For this review, take the finished solid that the model builds, in its own axes (mm). Face numbers are marked on the shaded views. A direction names the side the tool comes from. Coordinates: 2 decimals unless noted, no trailing zeros. Order: outer loops, then holes, each group sorted by start corner. A loop starts at its lowest first (then second) coordinate and runs counter-clockwise, first axis right, second up. Notation, with made-up numbers: (15.5, 71) - (27.5, 71) arc R24 cw to (27.5, 93) - close; hole circle Ø7 at (40, 58.5). An arc over 180 degrees is marked (long way). One line per item, written item: value. Start each with the question number.
(1) To check wall thickness, follow line 1 along Z through (x, y) = (190, -57); line 2 along X through (y, z) = (-8, 7); line 3 along Y through (x, z) = (220.5, 42.5). State the ranges of each line that lie inside material, in increasing order.
(2) Consider section C-C on z = 34. Write out the cut boundary in (x, y).
(3) Clearance check with flat-ended pins moving along their axes: pin 1 (4 mm diameter, centred on x = 156, y = 125, fed in from +Z); pin 2 (4 mm diameter, centred on x = 200.5, z = 49, fed in from +Y). State where each tip first meets the part, or that it passes through.
(4) Consider section D-D on y = 42. Write out the cut boundary in (x, z), then the cut area to 3 significant figures.
(5) Consider section B-B on x = 206. Write out the cut boundary in (y, z), then the cut area to 3 significant figures.
(6) Consider section A-A on y = 0. Write out the cut boundary in (x, z).
(7) For the marked faces 1, 2 and 3, list the 3-axis set-ups (+Z, -Z, +X, -X, +Y, -Y) from which the entire face can be reached by the end or side of a thin tool; tool diameter is ignored.
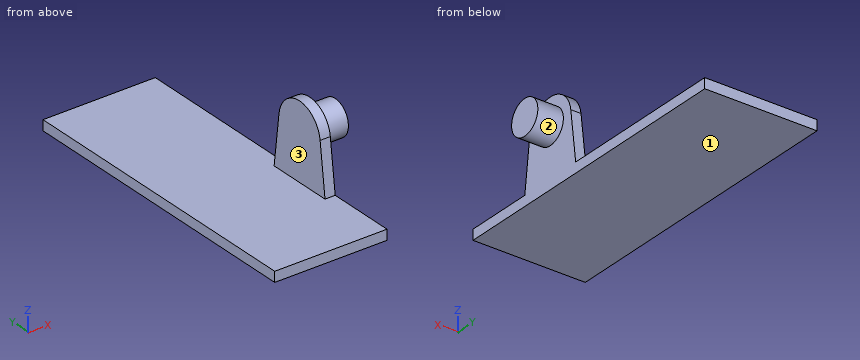
```python
from build123d import *

# Parameters (mm, degrees)
F4_W     = 110
F4_H     = 300
F5_DEPTH = 9.9999997765
F0_R     = 16.989496858
F1_DEPTH = 10
F2_DEPTH = 25


with BuildPart() as f5:
    # F4 (on Top) → F5 (new body)
    with BuildSketch(Plane.XY):
        with Locations((155, 50)):
            Rectangle(F4_W, F4_H)
    extrude(amount=-F5_DEPTH)

    # F0 (on face) → F1 (join)
    with BuildSketch(Plane.YZ.offset(210)):
        with BuildLine():
            ThreePointArc((26.601998421, 49.9582877529), (0, 73.3968899806), (-26.601998421, 49.9582877529))
            Line((-26.601998421, 49.9582877529), (-32.9437274149, 0))
            Line((-32.9437274149, 0), (32.9437274149, 0))
            Line((32.9437274149, 0), (26.601998421, 49.9582877529))
        make_face()
        with Locations((0, 46.5814173222)):
            Circle(F0_R, mode=Mode.SUBTRACT)
        with Locations((0, 46.5814173222)):
            Circle(F0_R)
    extrude(amount=-F1_DEPTH)

    # F0 (on face) → F2 (join)
    with BuildSketch(Plane.YZ.offset(210)):
        with Locations((0, 46.5814173222)):
            Circle(F0_R)
    extrude(amount=F2_DEPTH)


solid = f5.part
```
Geometry check:
1. line 1: z = -10 to 0
1. line 2: x = 200 to 210
1. line 3: y = -16.49 to 16.49
2. outline: (200, -28.63) - (210, -28.63) - (210, -11.42) - (235, -11.42) - (235, 11.42) - (210, 11.42) - (210, 28.63) - (200, 28.63) - close
3. pin 1: stops at z = 0
3. pin 2: stops at y = 26.98
4. outline: (100, -10) - (210, -10) - (210, 0) - (100, 0) - close
4. area: 1,100 mm^2
5. outline: (-100, -10) - (200, -10) - (200, 0) - (32.94, 0) - (26.6, 49.96) arc R26.82 ccw to (-26.6, 49.96) - (-32.94, 0) - (-100, 0) - close
5. area: 6,920 mm^2
6. outline: (100, -10) - (210, -10) - (210, 29.59) - (235, 29.59) - (235, 63.57) - (210, 63.57) - (210, 73.4) - (200, 73.4) - (200, 0) - (100, 0) - close
7. face 1: -Z, +X, -X, +Y, -Y
7. face 2: +X
7. face 3: +Z, -X, +Y, -Y
